Geometry check sheet. Reference: the model listing, model coordinates, mm. A direction names the side the tool comes from. Coordinates: 2 decimals unless noted, no trailing zeros. Write each loop counter-clockwise with the first axis right and the second up, starting at its lowest first coordinate (ties: lowest second). Pieces come first, ordered by that corner, then holes.
from build123d import *

# Parameters (mm, degrees)
F0_W     = 262.8
F0_H     = 148
F1_DEPTH = 50
F2_R     = 5
F3_R     = 5
F4_W     = 50
F4_H     = 40
F4_R     = 6.5
F5_DEPTH = 125


with BuildPart() as f1:
    # F0 (on Front) → F1 (new body)
    with BuildSketch(Plane.XZ):
        with Locations((75.004346, 56.001419)):
            Rectangle(F0_W, F0_H)
    extrude(amount=F1_DEPTH)

    # F2
    f2_edges = [f1.edges().sort_by_distance(p)[0] for p in [
        (206.404346, -25, -17.998581),
    ]]
    fillet(f2_edges, radius=F2_R)

    # F3
    f3_edges = [f1.edges().sort_by_distance(p)[0] for p in [
        (-56.395654, -25, -17.998581),
    ]]
    fillet(f3_edges, radius=F3_R)

    # F4 (on face) → F5 (cut)
    with BuildSketch(Plane.XY.offset(130.001419)):
        with Locations((-26.395654, -25)):
            Rectangle(F4_W, F4_H)
        with Locations((37.584728, -9.787194)):
            Circle(F4_R)
        with Locations((96.540727, -9.092722)):
            Circle(F4_R)
        with Locations((42.519221, -36.595406)):
            Circle(F4_R)
        with Locations((92.867015, -36.265045)):
            Circle(F4_R)
        with Locations((176.404346, -25)):
            Rectangle(F4_W, F4_H)
    extrude(amount=-F5_DEPTH, mode=Mode.SUBTRACT)


solid = f1.part
1. Sectioned sample at C-C, the plane z = 11.5. Record the boundary of the cut face in (x, y), and give its area (3 significant figures).
Computed values:
outline: (-56.4, -50) - (206.4, -50) - (206.4, 0) - (-56.4, 0) - close; hole (-51.4, -45) - (-1.4, -45) - (-1.4, -5) - (-51.4, -5) - close; hole circle Ø13 at (37.58, -9.79); hole circle Ø13 at (42.52, -36.6); hole circle Ø13 at (92.87, -36.27); hole circle Ø13 at (96.54, -9.09); hole (151.4, -45) - (201.4, -45) - (201.4, -5) - (151.4, -5) - close
area: 8,610 mm2
2. Thickness scan on line 1 along X through (y, z) = (-19, 107); line 2 along X through (y, z) = (-41, 110); line 3 along Y through (x, z) = (170.5, 28.5). Record the ranges inside material, lowest first.
Computed values:
line 1: x = -56.4 to -51.4, -1.4 to 151.4, 201.4 to 206.4
line 2: x = -56.4 to -51.4, -1.4 to 37.74, 47.3 to 88.41, 97.32 to 151.4, 201.4 to 206.4
line 3: y = -50 to -45, -5 to 0
3. Sectioned sample at D-D, the plane y = -13. Record the boundary of the cut face in (x, z), and give its area (3 significant figures).
Computed values:
outline: (-56.4, -13) arc R5 ccw to (-51.4, -18) - (201.4, -18) arc R5 ccw to (206.4, -13) - (206.4, 130) - (201.4, 130) - (201.4, 5) - (151.4, 5) - (151.4, 130) - (101.74, 130) - (101.74, 5) - (91.35, 5) - (91.35, 130) - (43.24, 130) - (43.24, 5) - (31.93, 5) - (31.93, 130) - (-1.4, 130) - (-1.4, 5) - (-51.4, 5) - (-51.4, 130) - (-56.4, 130) - close
area: 23,700 mm2
4. Access from +Z, -Z, +X, -X, +Y, -Y to the whole of each face (thin tool, end or side, straight path). Record for faces 4 (the flat face through (73, -50, 57)), 5 (the cylindrical face through (43.785, -7.835, 68.376)).
Computed values:
face 4: +Z, -Z, +X, -X, -Y
face 5: +Z
5. Gauge pin test, flat end, axial feed: pin 1 Ø6.5 at (x, y) = (39, -8.5) entering from +Z. Record the tip position at first contact, or that the pin passes through.
Computed values:
pin 1: stops at z = 5
6. Sectioned sample at B-B, the plane x = -15. Record the boundary of the cut face in (y, z).
Computed values:
outline: (-50, -18) - (0, -18) - (0, 130) - (-5, 130) - (-5, 5) - (-45, 5) - (-45, 130) - (-50, 130) - close
7. Draft check along X on faces 1 (the cylindrical face through (102.545, -11.582, 68.376)), 2 (the cylindrical face through (204.901, -25.35, -16.573)), 3 (the flat face through (73, 0, 57)). Enter one of: released by +X, released by -X, zero draft, split by the parting line, or undercut.
Computed values:
face 1: undercut
face 2: released by +X
face 3: zero draft
8. Sectioned sample at A-A, the plane y = -25. Record the boundary of the cut face in (x, z), and give its area (3 significant figures).
Computed values:
outline: (-56.4, -13) arc R5 ccw to (-51.4, -18) - (201.4, -18) arc R5 ccw to (206.4, -13) - (206.4, 130) - (201.4, 130) - (201.4, 5) - (151.4, 5) - (151.4, 130) - (-1.4, 130) - (-1.4, 5) - (-51.4, 5) - (-51.4, 130) - (-56.4, 130) - close
area: 26,400 mm2
